CAD build for the part. Positions are in the model's coordinates, mm. A direction names the side the tool comes from. Give positions to 0.01 mm unless a question says otherwise; leave off trailing zeros. Put each result on its own line as item: value. Start each with the question number.
1. Mould opens along Z. For faces 3 (the flat face through (68, 18, 0)), 4 (the flat face through (68, 18, -48)), 5 (the flat face through (68, 0, -24)), 6 (the flat face through (3, 2, -3.374)) say: +Z half, -Z half, draft (parallel to the pull), parting line (faces both ways), or undercut.
2. Tool access for faces 1 (the flat face through (5.121, 2, -8)), 2 (the flat face through (138, 18, -24)): list every direction of +Z, -Z, +X, -X, +Y, -Y with a clear straight run to the whole face (end or side of a thin tool).
3. Drop flat-ended pins along their axis: pin 1 (2 mm diameter, centred on y = 2.5, z = -6, fed in from -X); pin 2 (4 mm diameter, centred on x = 3, z = -6, fed in from -Y). Give the stop position or say it passes through.
from build123d import *

# Parameters (mm, degrees)
SKETCH1_W           = 138
SKETCH1_H           = 36
BOSS_EXTRUDE1_DEPTH = 48
FILLET2_R           = 1
SKETCH2_W           = 5.121114637
SKETCH2_H           = 9.72723973
CUT_EXTRUDE1_DEPTH  = 4


with BuildPart() as part:
    # Sketch1 → Boss-Extrude1 (new body)
    with BuildSketch(Plane.XY):
        with Locations((69, 18)):
            Rectangle(SKETCH1_W, SKETCH1_H)
    extrude(amount=-BOSS_EXTRUDE1_DEPTH)

    # Fillet2
    fillet2_edges = [part.edges().sort_by_distance(p)[0] for p in [
        (69, 36, -48),
        (69, 36, 0),
        (69, 0, 0),
        (69, 0, -48),
    ]]
    fillet(fillet2_edges, radius=FILLET2_R)

    # Sketch2 → Cut-Extrude1 (cut)
    with BuildSketch(Plane.XZ):
        with Locations((2.560557319, -8.237193023)):
            Rectangle(SKETCH2_W, SKETCH2_H)
    extrude(amount=-CUT_EXTRUDE1_DEPTH, mode=Mode.SUBTRACT)


solid = part.part
Report:
1. face 3: +Z half
1. face 4: -Z half
1. face 5: draft
1. face 6: undercut
2. face 1: -X, -Y
2. face 2: +Z, -Z, +X, +Y, -Y
3. pin 1: stops at x = 5.12
3. pin 2: stops at y = 4
